from build123d import *

# Parameters (mm, degrees)
BOSS_EXTRUDE1_DEPTH = 10
CUT_EXTRUDE36_DEPTH = 10


with BuildPart() as part:
    # Sketch1 → Boss-Extrude1 (new body)
    with BuildSketch(Plane.XY):
        with BuildLine():
            Line((-50, 60), (50, 60))
            ThreePointArc((50, 60), (57.071067812, 57.071067812), (60, 50))
            Line((60, 50), (60, -50))
            ThreePointArc((60, -50), (57.071067812, -57.071067812), (50, -60))
            Line((50, -60), (-50, -60))
            ThreePointArc((-50, -60), (-57.071067812, -57.071067812), (-60, -50))
            Line((-60, -50), (-60, 50))
            ThreePointArc((-60, 50), (-57.071067812, 57.071067812), (-50, 60))
        make_face()
    extrude(amount=BOSS_EXTRUDE1_DEPTH)

    # Sketch2 → Cut-Extrude36 (cut)
    with BuildSketch(Plane.XY.offset(10)):
        Polygon((-47.294871795, 50), (-31.729967949, 50), (-20.371794872, -13.842147436), (-7.851762821, 50), (8.193910256, 50), (20.653846154, -13.842147436), (31.991987179, 50), (47.576923077, 50), (29.80849359, -50), (12.761217949, -50), (0.141025641, 14.643429487), (-12.539262821, -50), (-29.506410256, -50), align=None)
    extrude(amount=-CUT_EXTRUDE36_DEPTH, mode=Mode.SUBTRACT)


solid = part.part
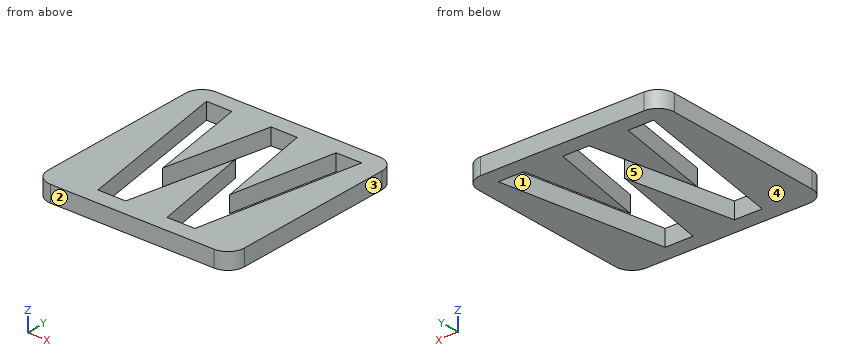
Could you check a few things on this model? Use its own coordinates, in mm. Face numbers are marked on the shaded views. A direction names the side the tool comes from. Round coordinates to 2 decimals unless told otherwise and drop trailing zeros. Loops run counter-clockwise (first coordinate to the right, second up) from the corner with the lowest first, then second, coordinate; pieces in that order, holes last. Notation, with made-up numbers: (68.5, -27) - (115.5, -27) arc R31 ccw to (115.5, 3) - close; hole circle Ø3 at (56, 3.5). An arc over 180 degrees is marked (long way). Write item = value, one per line.
1) Imagine slicing it at B-B (y = 0). Please give me the cut outline in (x, z), and give its area (3 significant figures).
Computed:
outline = (-60, 0) - (-38.4, 0) - (-38.4, 10) - (-60, 10) - close; (-22.83, 0) - (-17.66, 0) - (-17.66, 10) - (-22.83, 10) - close; (-2.73, 0) - (3, 0) - (3, 10) - (-2.73, 10) - close; (17.95, 0) - (23.11, 0) - (23.11, 10) - (17.95, 10) - close; (38.69, 0) - (60, 0) - (60, 10) - (38.69, 10) - close
area = 590 mm2
2) I'm going to push a flat-ended pin straight in: P1, Ø2, axis at x = -34.5, y = -11.5, coming from the +Z side. Where does the tip first touch, or does it pass through?
Computed:
P1 = through
3) If we mould it in two halves opening along X, with no side actions, what happens to the marked faces 3, 4 and 5? For each: pulls with the +X half, pulls with the -X half, needs draft (parallel to the pull), parting line crosses it, or undercut.
Computed:
face_3 = pulls with the +X half
face_4 = needs draft
face_5 = undercut
4) On a 3-axis mill with a long thin cutter (end or side, diameter ignored), from which of +Z, -Z, +X, -X, +Y, -Y can I reach the whole of each face in a straight line? I mean the marked faces 1 and 2. Say none if no direction works.
Computed:
face_1 = +Z, -Z
face_2 = +Z, -Z, +X, -X, -Y
5) I need wall thicknesses on line 1 along X through (y, z) = (-13, 2.5); line 2 along X through (y, z) = (-34, 6.5); line 3 along X through (y, z) = (46, 7.5). Which ranges of each line are inside material? Lowest first, please. Write a range as from..to.
Computed:
line_1 = -60..-36.09, -20.52..-20.21, -5.28..5.54, 20.49..20.8, 36.38..60
line_2 = -60..-32.35, -9.4..9.64, 32.65..60
line_3 = -60..-46.58, -31.02..-8.64, 8.97..31.28, 46.87..60
6) Imagine slicing it at D-D (y = -25.5). Please give me the cut outline in (x, z).
Computed:
outline = (-60, 0) - (-33.86, 0) - (-33.86, 10) - (-60, 10) - close; (-7.73, 0) - (7.98, 0) - (7.98, 10) - (-7.73, 10) - close; (34.16, 0) - (60, 0) - (60, 10) - (34.16, 10) - close
7) Imagine slicing it at A-A (z = 6.5). Please give me the cut outline in (x, y), and give its area (3 significant figures).
Computed:
outline = (-60, -50) arc R10 ccw to (-50, -60) - (50, -60) arc R10 ccw to (60, -50) - (60, 50) arc R10 ccw to (50, 60) - (-50, 60) arc R10 ccw to (-60, 50) - close; hole (-47.29, 50) - (-29.51, -50) - (-12.54, -50) - (0.14, 14.64) - (12.76, -50) - (29.81, -50) - (47.58, 50) - (31.99, 50) - (20.65, -13.84) - (8.19, 50) - (-7.85, 50) - (-20.37, -13.84) - (-31.73, 50) - close
area = 8,940 mm2
8) Imagine slicing it at C-C (x = -26.5). Please give me the cut outline in (y, z), and give its area (3 significant figures).
Computed:
outline = (-60, 0) - (-50, 0) - (-50, 10) - (-60, 10) - close; (20.6, 0) - (60, 0) - (60, 10) - (20.6, 10) - close
area = 494 mm2
